Part model, mm, in its own coordinate system. Coordinates: 2 decimals unless noted, no trailing zeros. Write each loop counter-clockwise with the first axis right and the second up, starting at its lowest first coordinate (ties: lowest second). Pieces come first, ordered by that corner, then holes. Notation, with made-up numbers: (2.25, 36) -> (14.25, 36) arc R4 cw to (14.25, 43) -> close; hole circle Ø5 at (80, 55). An arc over 180 degrees is marked (long way). Write item = value, one per line. Start each with the question number.
Q1. Band-saw the part on C-C, the plane z = 0.75. Give the number of separate pieces and of enclosed holes in the cut face, plus the area to 3 significant figures.
Q2. Probe line 1 (X direction, y = 0.55, z = -0.4); line 2 (Z direction, x = -3, y = -0.35); line 3 (X direction, y = -1.35, z = 0.55). List the from-to ranges inside material, lowest first.
Q3. Pin check, flat tip, straight feed: P1, Ø2, axis at y = -1, z = 2, coming from the +X side. Stop position of the tip, or through.
Q4. Band-saw the part on A-A, the plane y = -1.1. List the corners of the cut face in (x, z), plus the area to 3 significant figures.
Q5. Pull direction Z, two halves, no side cores. Call faces 1 (the cylindrical face through (-1.81, 0.03, -0.38)), 2 (the flat face through (-2, 0, 2.5)), 3 (the flat face through (-1.4, -2.5, -1.3)), 4 (the flat face through (-2, 0, -2.5)): released by +Z, released by -Z, zero draft, split by the parting line, or undercut.
Q6. Band-saw the part on B-B, the plane x = 0. List the corners of the cut face in (y, z), plus the area to 3 significant figures.
Solid Edge part; units mm, degrees
sketch "Sketch1" plane through (0, 0, 0) normal (0, -1, 0) x (1, 0, 0)
  circle A0 centre (0, 0) radius 1.25
  circle A1 centre (3, 0) radius 1.25
  circle A2 centre (-3, 0) radius 1.25
  circle A3 centre (-6, 0) radius 1.25
  line L0 (-6, 2.5) -> (3, 2.5)
  line L1 (5.5, 0) -> (5.5, -2.5)
  line L2 (3, -2.5) -> (5.5, -2.5)
  line L3 (3, -2.5) -> (-6, -2.5)
  line L4 (-6, -2.5) -> (-8.5, -2.5)
  line L5 (-8.5, 0) -> (-8.5, -2.5)
  arc A4 (-8.5, 0) -> (-6, 2.5) centre (-6, 0) cw
  arc A5 (3, 2.5) -> (5.5, 0) centre (3, 0) cw
extrude "Protrusion1" add sketch "Sketch1" along normal mid plane 5
fillet "Verrundung_1" radius 0.5 10 edges at (-1.5, -2.5, 2.5) (4.7678, -2.5, 1.7678) (5.5, -2.5, -1.25) (-7.7678, -2.5, 1.7678) (-8.5, -2.5, -1.25) (-1.5, 2.5, 2.5) (4.7678, 2.5, 1.7678) (5.5, 2.5, -1.25) (-7.7678, 2.5, 1.7678) (-8.5, 2.5, -1.25)
chamfer "Fase_1" distance 0.25 angle 45 8 edges at (-7.25, -2.5, 0) (-4.25, -2.5, 0) (-1.25, -2.5, 0) (1.75, -2.5, 0) (1.75, 2.5, 0) (-1.25, 2.5, 0) (-4.25, 2.5, 0) (-7.25, 2.5, 0)
Ans:
q1.separate_pieces = 5
q1.enclosed_holes = 0
q1.area = 28.0 mm2
q2.line_1 = -8.5 to -7.18, -4.82 to -4.18, -1.82 to -1.18, 1.18 to 1.82, 4.18 to 5.5
q2.line_2 = -2.5 to -1.25, 1.25 to 2.5
q2.line_3 = -8.44 to -7.12, -4.88 to -4.12, -1.88 to -1.12, 1.12 to 1.88, 4.12 to 5.44
q3.P1 = 5.29
q4.outline = (-8.5, -2.5) -> (5.5, -2.5) -> (5.5, 0) arc R2.5 ccw to (3, 2.5) -> (-6, 2.5) arc R2.5 ccw to (-8.5, 0) -> close; hole circle Ø2.5 at (-6, 0); hole circle Ø2.5 at (-3, 0); hole circle Ø2.5 at (0, 0); hole circle Ø2.5 at (3, 0)
q4.area = 47.7 mm2
q5.face_1 = undercut
q5.face_2 = released by +Z
q5.face_3 = zero draft
q5.face_4 = released by -Z
q6.outline = (-2.5, -2.5) -> (2.5, -2.5) -> (2.5, -1.5) -> (2.25, -1.25) -> (-2.25, -1.25) -> (-2.5, -1.5) -> close; (-2.5, 1.5) -> (-2.25, 1.25) -> (2.25, 1.25) -> (2.5, 1.5) -> (2.5, 2) arc R0.5 ccw to (2, 2.5) -> (-2, 2.5) arc R0.5 ccw to (-2.5, 2) -> close
q6.area = 12.3 mm2
